Here's how the part is built. I have some questions about the finished solid (model axes, mm). A direction names the side the tool comes from. Give positions to 0.01 mm unless a question says otherwise; leave off trailing zeros. Loops run counter-clockwise (first coordinate to the right, second up) from the corner with the lowest first, then second, coordinate; pieces in that order, holes last. Notation, with made-up numbers: (-7, -6.5) -> (-3, -6.5) arc R21 cw to (-3, 10.5) -> close; hole circle Ø7 at (-11, 3.5). An arc over 180 degrees is marked (long way). Answer in a Markdown table with one row per item. Add a question column.
Item 1: We'd pull the mould along X, two halves only. Please class faces 1 (the face through (-46.163, 111.698, 0.177)), 2 (the face through (1, 112, 8.065)), 3 (the face through (-42.948, 111.698, 0.637)), 4 (the face through (22.3, 60.01, 6.78)): released by +X, released by -X, zero draft, split by the parting line, or undercut.
Item 2: For P1, Ø2, axis at y = 46, z = 7, coming from the +X side; P2, Ø1.2, axis at x = -28, y = 65, coming from the +Z side; P3, Ø4, axis at y = 203, z = -4, coming from the +X side; P4, Ø6, axis at x = -38.1, z = 0, coming from the -Y side, each with a flat end and sliding along its axis, tell me the tip position at first contact or that it passes through.
Item 3: If we section it at C-C (y = 52): Write out the boundary of the cut face in (x, z), then the cut area to 3 significant figures.
Item 4: Which directions (+Z, -Z, +X, -X, +Y, -Y) give clear straight access to the entire face, cutting with the end or side of a thin tool? Please do faces 5 (the face through (14.831, 28.284, 6.777)), 6 (the face through (-30.48, 88.02, -0.11)), 7 (the face through (1, 226.568, 0)).
Item 5: If I drill on line 1 (X direction, y = 98, z = 0.5); line 2 (X direction, y = 146, z = 3.5); line 3 (Y direction, x = -24.5, z = 0), over which ranges is the centre line in solid material (lowest first)?
Item 6: If we section it at A-A (y = 204): Write out the boundary of the cut face in (x, z), then the cut area to 3 significant figures.
Item 7: If we section it at B-B (z = -2.75): Write out the boundary of the cut face in (x, y).
```python
from build123d import *

# Parameters (mm, degrees)
SKETCH1_R               = 4.8895
BOSS_EXTRUDE1_DEPTH     = 226.568
CUT_EXTRUDE2_DEPTH      = 232.785168476
CUT_EXTRUDE2_DEPTH_BACK = 232.785168476
CUT_EXTRUDE3_START      = 5.5245
CUT_EXTRUDE3_DEPTH      = 2.54
CUT_EXTRUDE4_DEPTH      = 232.785168476
CUT_EXTRUDE4_DEPTH_BACK = 8.0645
SKETCH6_R               = 1.5
SKETCH7_R               = 1.25
CUT_EXTRUDE5_DEPTH      = 8.0645


# Read off the part's stored shape, not the designer's step: Cut-Extrude3
with BuildPart() as part:
    # Sketch1 → Boss-Extrude1 (new body)
    with BuildSketch(Plane(origin=(0, 0, 0), x_dir=(1, 0, 0), z_dir=(0, 1, 0))):
        with BuildLine():
            Line((-38.1, 8.0645), (38.1, 8.0645))
            ThreePointArc((38.1, 8.0645), (46.1645, 0), (38.1, -8.0645))
            Line((38.1, -8.0645), (-38.1, -8.0645))
            ThreePointArc((-38.1, -8.0645), (-46.1645, 0), (-38.1, 8.0645))
        make_face()
        with Locations(Location((38.1, 0, 0), (0, 0, 270))):
            Circle(SKETCH1_R, mode=Mode.SUBTRACT)
        with Locations(Location((-38.1, 0, 0), (0, 0, 90))):
            Circle(SKETCH1_R, mode=Mode.SUBTRACT)
    extrude(amount=BOSS_EXTRUDE1_DEPTH)

    # Sketch2 → Cut-Extrude2 (cut, two sides: drawn at the far end of the back side and taken through both)
    with BuildSketch(Plane.XY.offset(8.0645).offset(-CUT_EXTRUDE2_DEPTH_BACK)):
        with BuildLine():
            Line((-24.13, 81.534), (-11.43, 81.534))
            ThreePointArc((-11.43, 81.534), (-5.08, 87.884), (-11.43, 94.234))
            Line((-11.43, 94.234), (-24.13, 94.234))
            ThreePointArc((-24.13, 94.234), (-30.48, 87.884), (-24.13, 81.534))
        make_face()
    extrude(amount=CUT_EXTRUDE2_DEPTH + CUT_EXTRUDE2_DEPTH_BACK, mode=Mode.SUBTRACT)

    # Cut-Extrude3 outline → Cut-Extrude3 (cut)
    with BuildSketch(Plane.XY.offset(CUT_EXTRUDE3_START)):
        Polygon((4.712362594, 41.284608988), (9.865946199, 35.669510433), (12.274110435, 35.669510433), (12.274110435, 31.069950753), (17.460700987, 25.418889406), (26.818871611, 25.418889406), (31.966756262, 31.069950753), (31.966756262, 49.931639685), (26.818871611, 49.931639685), (27.068707369, 32.39069939), (25.865559638, 31.069950753), (18.910545355, 31.069950753), (17.460700987, 32.39069939), (17.460700987, 35.669510433), (19.669379675, 35.669510433), (24.861712029, 41.369363995), (24.861712029, 57.217602301), (19.669379675, 62.874919643), (9.865946199, 62.874919643), (4.712362594, 57.217602301), align=None)
        Polygon((17.460700987, 41.284608988), (17.460700987, 49.931639685), (12.274110435, 49.931639685), (12.274110435, 41.284608988), (11.176923497, 41.284608988), (9.865946199, 42.595586286), (9.865946199, 55.774170995), (11.176923497, 57.217602301), (18.57945551, 57.217602301), (19.669379675, 55.774170995), (19.669379675, 42.595586286), (18.57945551, 41.284608988), align=None, mode=Mode.SUBTRACT)
    extrude(amount=CUT_EXTRUDE3_DEPTH, mode=Mode.SUBTRACT)

    # Sketch6 → Cut-Extrude4 (cut, two sides: drawn at the far end of the back side and taken through both)
    with BuildSketch(Plane.XY.offset(8.0645).offset(-CUT_EXTRUDE4_DEPTH_BACK)):
        with Locations(Location((28.3845, 175.768, 0), (0, 0, 180))):
            Circle(SKETCH6_R)
        with Locations(Location((5.9595, 175.768, 0), (0, 0, 180))):
            Circle(SKETCH6_R)
        with Locations(Location((5.9595, 83.743, 0), (0, 0, 180))):
            Circle(SKETCH6_R)
        with Locations(Location((28.3845, 83.743, 0), (0, 0, 180))):
            Circle(SKETCH6_R)
    extrude(amount=CUT_EXTRUDE4_DEPTH + CUT_EXTRUDE4_DEPTH_BACK, mode=Mode.SUBTRACT)

    # Sketch7 → Cut-Extrude5 (cut)
    with BuildSketch(Plane.XY.offset(8.0645)):
        with Locations((-12.3825, 64.516)):
            Circle(SKETCH7_R)
        with Locations((-28.3845, 64.516)):
            Circle(SKETCH7_R)
        with Locations((-12.3825, 19.05)):
            Circle(SKETCH7_R)
        with Locations((-28.3845, 19.05)):
            Circle(SKETCH7_R)
    extrude(amount=-CUT_EXTRUDE5_DEPTH, mode=Mode.SUBTRACT)


solid = part.part
```
Recorded:
| question | item | result |
|---|---|---|
| 1 | face 1 | released by -X |
| 1 | face 2 | zero draft |
| 1 | face 3 | undercut |
| 1 | face 4 | undercut |
| 2 | P1 | stops at x = 43.49 |
| 2 | P2 | stops at z = 0 |
| 2 | P3 | stops at x = 45.91 |
| 2 | P4 | passes through |
| 3 | outline | (-38.1, -8.06) -> (38.1, -8.06) arc R8.06 ccw to (38.1, 8.06) -> (24.86, 8.06) -> (24.86, 5.52) -> (19.67, 5.52) -> (19.67, 8.06) -> (9.87, 8.06) -> (9.87, 5.52) -> (4.71, 5.52) -> (4.71, 8.06) -> (-38.1, 8.06) arc R8.06 ccw to start; hole circle Ø9.78 at (-38.1, 0); hole circle Ø9.78 at (38.1, 0) |
| 3 | area | 1,260 mm^2 |
| 4 | face 5 | +Z |
| 4 | face 6 | +Z, -Z |
| 4 | face 7 | +Z, -Z, +X, -X, +Y |
| 5 | line 1 | x = -46.15 to -42.96, -33.24 to 33.24, 42.96 to 46.15 |
| 5 | line 2 | x = -45.37 to -41.51, -34.69 to 34.69, 41.51 to 45.37 |
| 5 | line 3 | y = 0 to 81.54, 94.22 to 226.57 |
| 6 | outline | (-38.1, -8.06) -> (38.1, -8.06) arc R8.06 ccw to (38.1, 8.06) -> (-38.1, 8.06) arc R8.06 ccw to start; hole circle Ø9.78 at (-38.1, 0); hole circle Ø9.78 at (38.1, 0) |
| 6 | area | 1,280 mm^2 |
| 7 | outline | (-45.68, 0) -> (-42.14, 0) -> (-42.14, 226.57) -> (-45.68, 226.57) -> close; (-34.06, 0) -> (34.06, 0) -> (34.06, 226.57) -> (-34.06, 226.57) -> close; (42.14, 0) -> (45.68, 0) -> (45.68, 226.57) -> (42.14, 226.57) -> close; hole (-24.13, 81.53) -> (-11.43, 81.53) arc R6.35 ccw to (-11.43, 94.23) -> (-24.13, 94.23) arc R6.35 ccw to start |
